Here's the drawing with two shaded views (mm, measured from the low corner). I have some questions. A direction names the side the tool comes from. Give positions to 0.01 mm unless a question says otherwise; leave off trailing zeros. Loops run counter-clockwise (first coordinate to the right, second up) from the corner with the lowest first, then second, coordinate; pieces in that order, holes last. Notation, with made-up numbers: (81, 41.5) - (116, 41.5) arc R36 ccw to (116, 75.5) - close; hole circle Ø1 at (76.5, -25.75). An arc over 180 degrees is marked (long way). Answer as a JSON object with one key per item and string values. Group by question number.
Item 1: Will these pins go through, and if not, where does the flat tip stop? pin 1 (4 mm diameter, centred on x = 19.5, z = 23.5, fed in from +Y); pin 2 (5 mm diameter, centred on x = 14.5, z = 15, fed in from +Y); pin 3 (3 mm diameter, centred on x = 30.5, y = 9, fed in from +Z).
Item 2: Thinking about a two-plate mould opening in X: for the marked faces 4, 5, 6 and 7, which applies, pulls with the +X half, pulls with the -X half, needs draft (parallel to the pull), parting line crosses it, or undercut?
Item 3: Suppose I cut it at B-B on y = 9. Count the separate pieces of the cut face and the enclosed holes in it, and give its area (3 significant figures).
Item 4: Please list where these lines run through material, in increasing order: L1, parallel to Z at x = 49.5, y = 6.5; L2, parallel to Z at x = 58, y = 13.25; L3, parallel to Z at x = 45.5, y = 5.25.
Item 5: Suppose I cut it at D-D on x = 5. Write out the boundary of the cut face in (y, z), and give its area (3 significant figures).
Item 6: Suppose I cut it at C-C on z = 20.5. Write out the boundary of the cut face in (x, y), and give its area (3 significant figures).
Item 7: Which directions (+Z, -Z, +X, -X, +Y, -Y) give clear straight access to the entire face, cutting with the end or side of a thin tool? Please do the marked faces 1, 2 and 3.
Item 8: Suppose I cut it at A-A on x = 62.5. Write out the boundary of the cut face in (y, z).
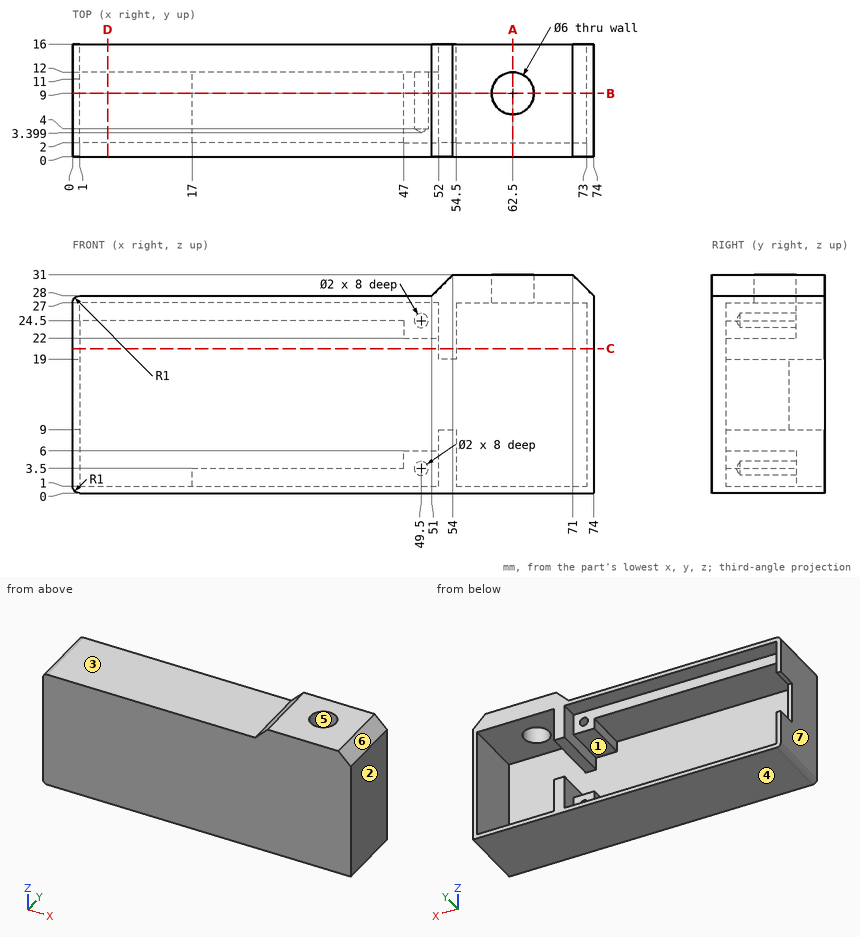
Worked out:
{
 "1": {"pin 1": "stops at y = 12", "pin 2": "stops at y = 2", "pin 3": "stops at z = 28"},
 "2": {"face 4": "needs draft", "face 5": "undercut", "face 6": "pulls with the +X half", "face 7": "pulls with the -X half"},
 "3": {"separate pieces": "1", "enclosed holes": "2", "area": "509 mm2"},
 "4": {"L1": "z = 0 to 2.5, 4.5 to 6, 22 to 23.5, 25.5 to 28", "L2": "z = 0 to 1, 27 to 31", "L3": "z = 0 to 3.5, 24.5 to 28"},
 "5": {"outline": "(0, 0) - (16, 0) - (16, 1) - (2, 1) - (2, 24.5) - (12, 24.5) - (12, 27) - (16, 27) - (16, 28) - (0, 28) - close", "area": "109 mm2"},
 "6": {"outline": "(0, 0) - (74, 0) - (74, 16) - (73, 16) - (73, 2) - (54.5, 2) - (54.5, 16) - (52, 16) - (52, 2) - (1, 2) - (1, 16) - (0, 16) - close", "area": "211 mm2"},
 "7": {"face 1": "+Y", "face 2": "+Z, -Z, +X, +Y, -Y", "face 3": "+Z, -X, +Y, -Y"},
 "8": {"outline": "(0, 0) - (16, 0) - (16, 1) - (2, 1) - (2, 27) - (6, 27) - (6, 31) - (0, 31) - close; (12, 27) - (16, 27) - (16, 31) - (12, 31) - close"}
}
